from build123d import *

# Parameters (mm, degrees)
PLASTIC_DEPTH = 2.54
SKETCH2_W     = 11.44
SKETCH2_H     = 0.6
CONTACT_DEPTH = 0.3
CHAMFER1_SIZE = 0.1


with BuildPart() as part:
    # Sketch1 → Plastic (new body)
    with BuildSketch(Plane.XY):
        Polygon((-0.77, 1.27), (0.77, 1.27), (1.27, 0.77), (1.27, -0.77), (0.77, -1.27), (-0.77, -1.27), (-1.27, -0.77), (-1.27, 0.77), align=None)
    extrude(amount=PLASTIC_DEPTH)

    # Sketch2 → Contact (add, symmetric)
    with BuildSketch(Plane(origin=(0, 0, 0), x_dir=(0, 0, -1), z_dir=(1, 0, 0))):
        with Locations((-3.18, 0)):
            Rectangle(SKETCH2_W, SKETCH2_H)
    extrude(amount=CONTACT_DEPTH, both=True)

    # Chamfer1
    chamfer1_edges = [part.edges().sort_by_distance(p)[0] for p in [
        (0, -0.3, 8.9),
        (0.3, 0, 8.9),
        (-0.3, 0, -2.54),
        (0, -0.3, -2.54),
        (0, 0.3, -2.54),
        (-0.3, 0, 8.9),
        (0, 0.3, 8.9),
        (0.3, 0, -2.54),
    ]]
    chamfer(chamfer1_edges, length=CHAMFER1_SIZE)


solid = part.part
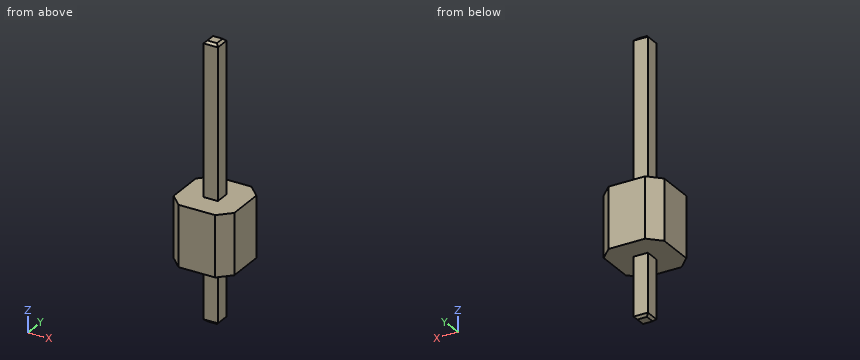
CAD build for the part. Positions are in the model's coordinates, mm. Round coordinates to 2 decimals unless told otherwise and drop trailing zeros. Write each loop counter-clockwise with the first axis right and the second up, starting at its lowest first coordinate (ties: lowest second). Pieces come first, ordered by that corner, then holes.
(1) Drop flat-ended pins along their axis: P1, Ø1.5, axis at x = 0.5, z = 6.5, coming from the +Y side; P2, Ø0.5, axis at y = 0, z = 7, coming from the -X side; P3, Ø0.7, axis at x = 0, z = -0.5, coming from the -Y side. Give the stop position or say it passes through.
(2) Slice it at D-D, the plane x = 0.9. Write the cut outline in (y, z), and give its area (3 significant figures).
(3) Slice it at A-A, the plane x = -0.1. Write the cut outline in (y, z).
(4) Slice it at C-C, the plane y = 0.95. Write the cut outline in (x, z).
(5) Probe line 1 along Z through (x, y) = (-0.7, -0.55); line 2 along Y through (x, z) = (0, 4.75). List the from-to ranges inside material, lowest first.
(6) Slice it at B-B, the plane z = 1. Write the cut outline in (x, y), and give its area (3 significant figures).
From the geometry:
1. P1: stops at y = 0.3
1. P2: stops at x = -0.3
1. P3: stops at y = -0.3
2. outline: (-1.14, 0) - (1.14, 0) - (1.14, 2.54) - (-1.14, 2.54) - close
2. area: 5.79 mm2
3. outline: (-1.27, 0) - (-0.3, 0) - (-0.3, -2.44) - (-0.2, -2.54) - (0.2, -2.54) - (0.3, -2.44) - (0.3, 0) - (1.27, 0) - (1.27, 2.54) - (0.3, 2.54) - (0.3, 8.8) - (0.2, 8.9) - (-0.2, 8.9) - (-0.3, 8.8) - (-0.3, 2.54) - (-1.27, 2.54) - close
4. outline: (-1.09, 0) - (1.09, 0) - (1.09, 2.54) - (-1.09, 2.54) - close
5. line 1: z = 0 to 2.54
5. line 2: y = -0.3 to 0.3
6. outline: (-1.27, -0.77) - (-0.77, -1.27) - (0.77, -1.27) - (1.27, -0.77) - (1.27, 0.77) - (0.77, 1.27) - (-0.77, 1.27) - (-1.27, 0.77) - close
6. area: 5.95 mm2
